The listing builds one solid part. Answer for the finished solid, in the listing's coordinates (mm). A direction names the side the tool comes from. Give positions to 0.01 mm unless a question says otherwise; leave off trailing zeros. Write each loop counter-clockwise with the first axis right and the second up, starting at its lowest first coordinate (ties: lowest second). Pieces come first, ordered by that corner, then holes. Notation, with made-up numbers: (76.5, 20) -> (95.5, 20) arc R28 ccw to (95.5, 41) -> close; hole circle Ø2 at (88, 38.5). An arc over 180 degrees is marked (long way). Put each result on its own line as item: value. Start each with the question number.
1) For faces 4 (the flat face through (0, 3.5, 6)), 5 (the flat face through (10.2, 0, 5)), 6 (the flat face through (-2.3, -4, 6)), determine the directions among +Z, -Z, +X, -X, +Y, -Y from which every point of the face is accessible in a straight line to the end or side of a thin tool.
2) A cutting plane is placed at B-B (y = -0.5). Write down the section's boundary in (x, z), then the cut area to 3 significant figures.
3) A cutting plane is placed at C-C (z = 8). Write down the section's boundary in (x, y).
4) A cutting plane is placed at D-D (x = 6.75). Write down the section's boundary in (y, z).
5) A cutting plane is placed at A-A (x = 1). Write down the section's boundary in (y, z), then the cut area to 3 significant figures.
6) A flat-ended cylindrical pin translates along its axis: pin 1 Ø4 at (x, y) = (0, 0) entering from +Z. Find the tip coordinate at first contact, or state that the pin passes through.
7) Find the intervals of material crossed by line 1 along Y through (x, z) = (-8, 6); line 2 along X through (y, z) = (-3, 8.5); line 3 along Z through (x, y) = (-3.25, -1.5), in increasing order. Write a range as from..to.
8) For a pull along X with two mould halves and no side action, classify faces 1 (the flat face through (0, 4.5, 5)), 2 (the flat face through (-9.2, 0, 6)), 3 (the flat face through (-10.2, 0, 5)) as released by +X, released by -X, zero draft, split by the parting line, or undercut.
from build123d import *

# Parameters (mm, degrees)
BOX004_W        = 4.6
BOX004_H        = 2
BOX004_DEPTH    = 6.65
BOX003_W        = 18
BOX003_H        = 7
BOX003_DEPTH    = 6.65
BOX002_W        = 20.4
BOX002_H        = 9
BOX002_DEPTH    = 9
CHAMFER001_SIZE = 0.3


with BuildPart() as cube004:
    # Box004 → Box004 (new body)
    with BuildSketch(Plane(origin=(-2.3, -5, 2.55), x_dir=(1, 0, 0), z_dir=(0, 0, 1))):
        with Locations((2.3, 1)):
            Rectangle(BOX004_W, BOX004_H)
    extrude(amount=BOX004_DEPTH)


with BuildPart() as cube003:
    # Box003 → Box003 (new body)
    with BuildSketch(Plane(origin=(-9.2, -3.5, 2.55), x_dir=(1, 0, 0), z_dir=(0, 0, 1))):
        with Locations((9, 3.5)):
            Rectangle(BOX003_W, BOX003_H)
    extrude(amount=BOX003_DEPTH)


with BuildPart() as chamfer001:
    # Box002 → Box002 (new body)
    with BuildSketch(Plane(origin=(-10.2, -4.5, 0.2), x_dir=(1, 0, 0), z_dir=(0, 0, 1))):
        with Locations((10.2, 4.5)):
            Rectangle(BOX002_W, BOX002_H)
    extrude(amount=BOX002_DEPTH)

    # Cut: cut Cube003
    add(cube003.part, mode=Mode.SUBTRACT)

    # Cut001: cut Cube004
    add(cube004.part, mode=Mode.SUBTRACT)

    # Chamfer001
    chamfer001_edges = [chamfer001.edges().sort_by_distance(p)[0] for p in [
        (5.55, -3.5, 9.2),
        (8.8, 0, 9.2),
        (-0.2, 3.5, 9.2),
        (-9.2, 0, 9.2),
        (-5.75, -3.5, 9.2),
    ]]
    chamfer(chamfer001_edges, length=CHAMFER001_SIZE)


solid = chamfer001.part
Reply:
1. face 4: +Z
1. face 5: +Z, -Z, +X, +Y, -Y
1. face 6: +Z, -Y
2. outline: (-10.2, 0.2) -> (10.2, 0.2) -> (10.2, 9.2) -> (9.1, 9.2) -> (8.8, 8.9) -> (8.8, 2.55) -> (-9.2, 2.55) -> (-9.2, 8.9) -> (-9.5, 9.2) -> (-10.2, 9.2) -> close
2. area: 63.8 mm2
3. outline: (-10.2, -4.5) -> (-2.3, -4.5) -> (-2.3, -3.5) -> (-9.2, -3.5) -> (-9.2, 3.5) -> (8.8, 3.5) -> (8.8, -3.5) -> (2.3, -3.5) -> (2.3, -4.5) -> (10.2, -4.5) -> (10.2, 4.5) -> (-10.2, 4.5) -> close
4. outline: (-4.5, 0.2) -> (4.5, 0.2) -> (4.5, 9.2) -> (3.8, 9.2) -> (3.5, 8.9) -> (3.5, 2.55) -> (-3.5, 2.55) -> (-3.5, 8.9) -> (-3.8, 9.2) -> (-4.5, 9.2) -> close
5. outline: (-4.5, 0.2) -> (4.5, 0.2) -> (4.5, 9.2) -> (3.8, 9.2) -> (3.5, 8.9) -> (3.5, 2.55) -> (-4.5, 2.55) -> close
5. area: 27.8 mm2
6. pin 1: stops at z = 2.55
7. line 1: y = -4.5..-3.5, 3.5..4.5
7. line 2: x = -10.2..-9.2, 8.8..10.2
7. line 3: z = 0.2..2.55
8. face 1: zero draft
8. face 2: undercut
8. face 3: released by -X
